Here's the drawing with two shaded views (mm, measured from the low corner). I have some questions. A direction names the side the tool comes from. Give positions to 0.01 mm unless a question says otherwise; leave off trailing zeros. Loops run counter-clockwise (first coordinate to the right, second up) from the corner with the lowest first, then second, coordinate; pieces in that order, holes last.
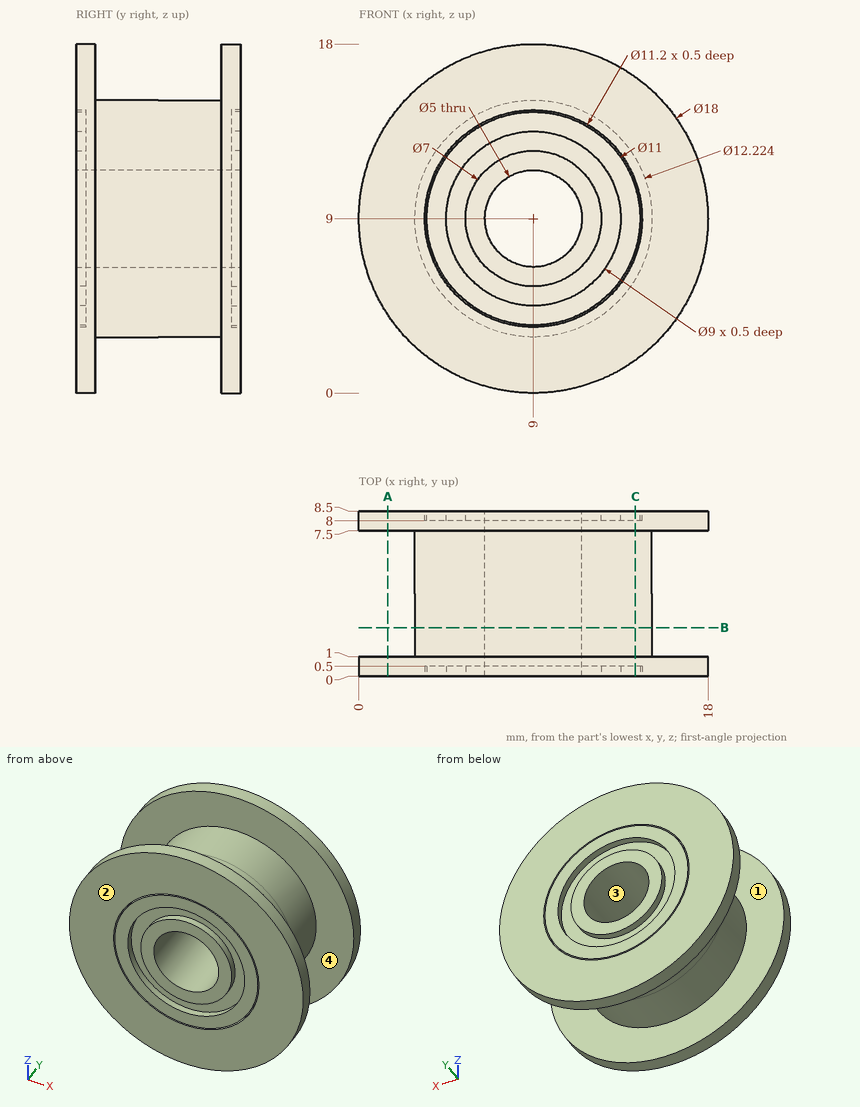
(1) Thinking about a two-plate mould opening in Z: for the marked faces 3 and 4, which applies, pulls with the +Z half, pulls with the -Z half, needs draft (parallel to the pull), parting line crosses it, or undercut?
Returned:
face 3: undercut
face 4: needs draft
(2) Suppose I cut it at B-B on y = 2.5. List the corners of the cut face in (x, z) for me (1 decimal).
Returned:
outline: circle Ø12.2 at (9, 9); hole circle Ø5 at (9, 9)
(3) Suppose I cut it at C-C on x = 14.25. List the corners of the cut face in (y, z) for me.
Returned:
outline: (0, 1.69) - (1, 1.69) - (1, 5.87) - (7.5, 5.87) - (7.5, 1.69) - (8.5, 1.69) - (8.5, 7.05) - (8, 7.05) - (8, 7.36) - (8.5, 7.36) - (8.5, 10.64) - (8, 10.64) - (8, 10.95) - (8.5, 10.95) - (8.5, 16.31) - (7.5, 16.31) - (7.5, 12.13) - (1, 12.13) - (1, 16.31) - (0, 16.31) - (0, 10.95) - (0.5, 10.95) - (0.5, 10.64) - (0, 10.64) - (0, 7.36) - (0.5, 7.36) - (0.5, 7.05) - (0, 7.05) - close
(4) Which directions (+Z, -Z, +X, -X, +Y, -Y) give clear straight access to the entire face, cutting with the end or side of a thin tool? Please do the marked faces 1 and 2.
Returned:
face 1: none
face 2: +Z, -Z, +X, -X, -Y
(5) Will these pins go through, and if not, where does the flat tip stop? P1, Ø2, axis at y = 2.5, z = 9, coming from the +X side; P2, Ø3, axis at y = 1.5, z = 13.5, coming from the -X side (1 decimal); P3, Ø4.5, axis at x = 9, z = 9, coming from the +Y side.
Returned:
P1: stops at x = 15.11
P2: stops at x = 0.5
P3: passes through
(6) Suppose I cut it at A-A on x = 1.5. List the corners of the cut face in (y, z) for me (1 decimal).
Returned:
outline: (0, 4) - (1, 4) - (1, 14) - (0, 14) - close; (7.5, 4) - (8.5, 4) - (8.5, 14) - (7.5, 14) - close
(7) Please list where these lines run through material, in increasing order: probe 1 along Y at (x, z) = (9, 2.75); probe 2 along X at (y, z) = (6.75, 9); probe 3 along Z at (x, y) = (10, 3.75).
Returned:
probe 1: y = 0 to 1, 7.5 to 8.5
probe 2: x = 2.89 to 6.5, 11.5 to 15.11
probe 3: z = 2.97 to 6.71, 11.29 to 15.03
